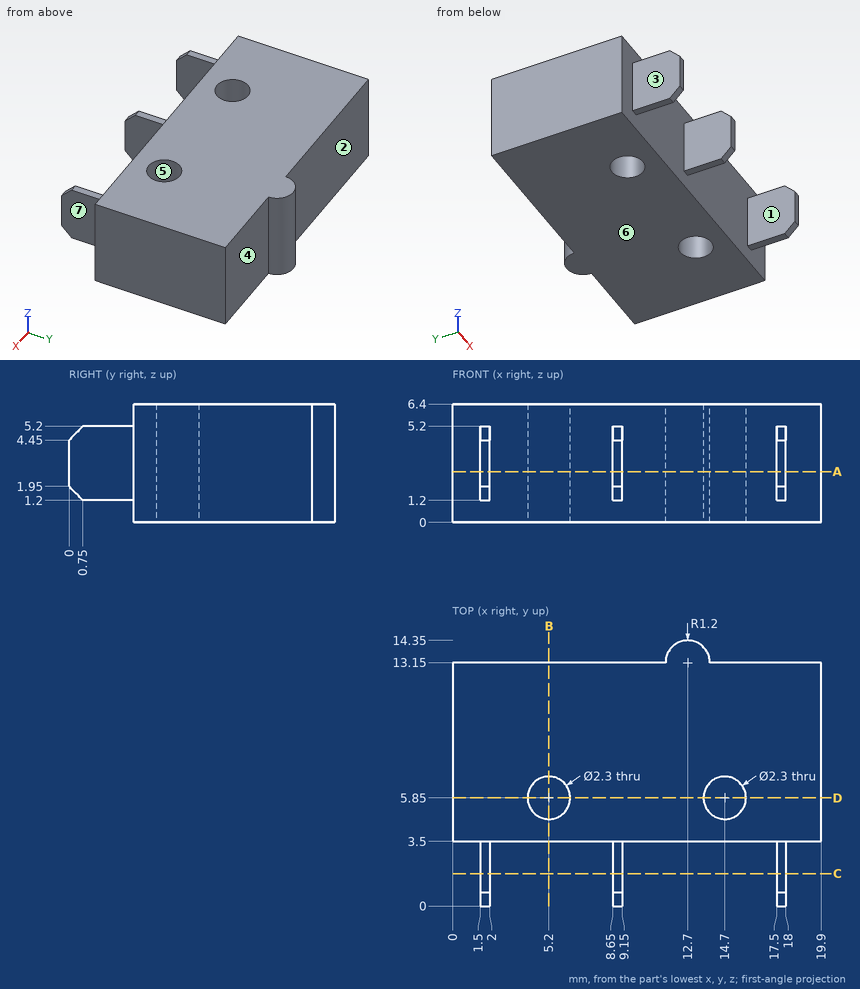
Design review of the part shown in the three views and the two pictorial views. Dimensions are in mm from the part's minimum x, y and z. A direction names the side the tool comes from. Coordinates: 2 decimals unless noted, no trailing zeros. Loops run counter-clockwise (first coordinate to the right, second up) from the corner with the lowest first, then second, coordinate; pieces in that order, holes last. Notation, with made-up numbers: M -14,60.5 L 14,60.5 A19 cw 14,76.5 Z; hole C -37,69.5 d4. An arc over 180 degrees is marked long. Put each result on its own line as item: value. Start each with the question number.
Q1. Add section D-D (y = 5.85). Write out the cut boundary in (x, z).
Q2. Clearance check with flat-ended pins moving along their axes: pin 1 (1.8 mm diameter, centred on y = 2.5, z = 3, fed in from -X); pin 2 (1 mm diameter, centred on y = 2.5, z = 2.5, fed in from +X); pin 3 (3 mm diameter, centred on x = 5, z = 1, fed in from +Y). State where each tip first meets the part, or that it passes through.
Q3. Add section B-B (x = 5.2). Write out the cut boundary in (y, z), and give its area (3 significant figures).
Q4. For the marked faces 1, 2, 3 and 4, list the 3-axis set-ups (+Z, -Z, +X, -X, +Y, -Y) from which the entire face can be reached by the end or side of a thin tool; tool diameter is ignored.
Q5. Wall thickness on line 1 (Y direction, x = 5.2, z = 1.5); line 2 (Y direction, x = 10, z = 6.25); line 3 (Y direction, x = 14.25, z = 2): over which ranges is each line inside the solid? List them lowest first.
Q6. Add section A-A (z = 2.75). Write out the cut boundary in (x, y).
Q7. The part is to be moulded in two halves that separate along X. For the marked faces 5, 6 and 7, say which applies: +X half, -X half, draft (parallel to the pull), parting line (faces both ways), or undercut.
Q8. Add section C-C (y = 1.75). Write out the cut boundary in (x, z).
Answers:
1. outline: M 0,0 L 4.05,0 L 4.05,6.4 L 0,6.4 Z; M 6.35,0 L 13.55,0 L 13.55,6.4 L 6.35,6.4 Z; M 15.85,0 L 19.9,0 L 19.9,6.4 L 15.85,6.4 Z
2. pin 1: stops at x = 1.5
2. pin 2: stops at x = 18
2. pin 3: stops at y = 13.15
3. outline: M 3.5,0 L 4.7,0 L 4.7,6.4 L 3.5,6.4 Z; M 7,0 L 13.15,0 L 13.15,6.4 L 7,6.4 Z
3. area: 47.0 mm^2
4. face 1: +Z, -Z, -Y
4. face 2: +Z, -Z, -X, +Y
4. face 3: +Z, -Z, -X, -Y
4. face 4: +Z, -Z, +X, +Y
5. line 1: y = 3.5 to 4.7, 7 to 13.15
5. line 2: y = 3.5 to 13.15
5. line 3: y = 3.5 to 4.79, 6.91 to 13.15
6. outline: M 0,3.5 L 1.5,3.5 L 1.5,0 L 2,0 L 2,3.5 L 8.65,3.5 L 8.65,0 L 9.15,0 L 9.15,3.5 L 17.5,3.5 L 17.5,0 L 18,0 L 18,3.5 L 19.9,3.5 L 19.9,13.15 L 13.9,13.15 A1.2 ccw 11.5,13.15 L 0,13.15 Z; hole C 5.2,5.85 d2.3; hole C 14.7,5.85 d2.3
7. face 5: undercut
7. face 6: draft
7. face 7: +X half
8. outline: M 1.5,1.2 L 2,1.2 L 2,5.2 L 1.5,5.2 Z; M 8.65,1.2 L 9.15,1.2 L 9.15,5.2 L 8.65,5.2 Z; M 17.5,1.2 L 18,1.2 L 18,5.2 L 17.5,5.2 Z
